Input: part model. Units: mm. Frame: model coordinates. Face numbers are marked on the shaded views. Coordinates: 2 decimals unless noted, no trailing zeros. Write each loop counter-clockwise with the first axis right and the second up, starting at its lowest first coordinate (ties: lowest second). Pieces come first, ordered by that corner, then holes.
1) Draft query along Z for the marked faces 1, 2, 3 and 4. Return one class per face: pulls with the +Z half, pulls with the -Z half, needs draft (parallel to the pull), parting line crosses it, or undercut.
2) Section query D-D (x = 35). Output: boundary loops of the cut face in (y, z), then the cut area to 3 significant figures.
3) Line query: L1, parallel to Z at x = 35, y = 0.2; L2, parallel to Z at x = -27, y = 10.5; L3, parallel to Z at x = -70, y = 0.6. Output: solid intervals per line, ascending.
4) Section query A-A (y = 16.75). Output: boundary loops of the cut face in (x, z), then the cut area to 3 significant figures.
5) Pin query (flat end, axial travel): pin 1 Ø4 at (x, z) = (-7, 0) entering from -Y; pin 2 Ø4 at (x, y) = (-23, 17) entering from +Z; pin 3 Ø0.5 at (x, y) = (-12.5, 0.5) entering from -Z; pin 4 Ø0.8 at (x, y) = (-20.5, 0.5) entering from +Z. Return the tip coordinate at first contact, or that it passes through.
6) Section query C-C (z = -40). Output: boundary loops of the cut face in (x, y), then the cut area to 3 significant figures.
7) Section query B-B (x = -7). Output: boundary loops of the cut face in (y, z), then the cut area to 3 significant figures.
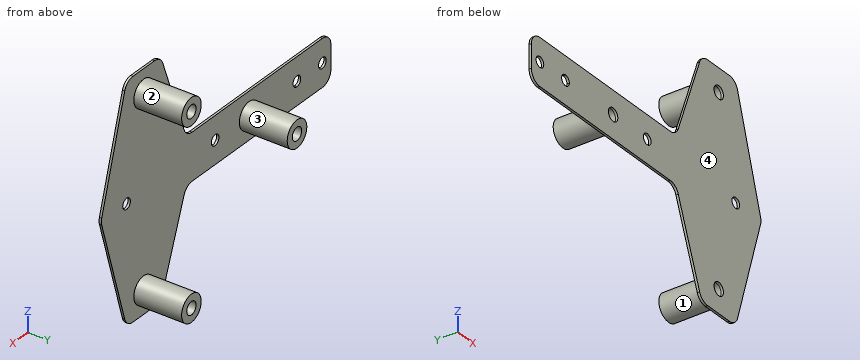
from build123d import *

# Parameters (mm, degrees)
BOSS_EXTRUDE1_DEPTH = 1
SKETCH2_R           = 2.75
CUT_EXTRUDE1_DEPTH  = 2
SKETCH3_R           = 5.75
SKETCH3_R_2         = 2.75
BOSS_EXTRUDE2_DEPTH = 20.5
SKETCH4_R           = 2.25
CUT_EXTRUDE2_DEPTH  = 2
SKETCH5_R           = 2.25
BOSS_EXTRUDE3_DEPTH = 1
SKETCH6_R           = 2.25
CUT_EXTRUDE3_DEPTH  = 2


with BuildPart() as part:
    # Sketch1 → Boss-Extrude1 (new body)
    with BuildSketch(Plane(origin=(0, 0, 0), x_dir=(1, 0, 0), z_dir=(0, 1, 0))):
        with BuildLine():
            Line((-55, 10), (6.534997659, 10))
            ThreePointArc((6.534997659, 10), (9.382971848, 10.890371912), (11.216643547, 13.244382792))
            Line((11.216643547, 13.244382792), (23.783356453, 46.755617208))
            ThreePointArc((23.783356453, 46.755617208), (25.617028152, 49.109628088), (28.465002341, 50))
            Line((28.465002341, 50), (41.279846746, 50))
            ThreePointArc((41.279846746, 50), (44.264499394, 49.011464641), (46.068978172, 46.436739428))
            Line((46.068978172, 46.436739428), (59.568978172, 1.436739428))
            ThreePointArc((59.568978172, 1.436739428), (59.779846746, 0), (59.568978172, -1.436739428))
            Line((59.568978172, -1.436739428), (46.068978172, -46.436739428))
            ThreePointArc((46.068978172, -46.436739428), (44.264499394, -49.011464641), (41.279846746, -50))
            Line((41.279846746, -50), (28.465002341, -50))
            ThreePointArc((28.465002341, -50), (25.617028152, -49.109628088), (23.783356453, -46.755617208))
            Line((23.783356453, -46.755617208), (11.216643547, -13.244382792))
            ThreePointArc((11.216643547, -13.244382792), (9.382971848, -10.890371912), (6.534997659, -10))
            Line((6.534997659, -10), (-55, -10))
            ThreePointArc((-55, -10), (-58.535533906, -8.535533906), (-60, -5))
            Line((-60, -5), (-60, 5))
            ThreePointArc((-60, 5), (-58.535533906, 8.535533906), (-55, 10))
        make_face()
    extrude(amount=BOSS_EXTRUDE1_DEPTH)

    # Sketch2 → Cut-Extrude1 (cut, through all)
    with BuildSketch(Plane(origin=(0, 1, 0), x_dir=(1, 0, 0), z_dir=(0, 1, 0))):
        with Locations((-27, 0)):
            Circle(SKETCH2_R)
        with Locations((35, 40)):
            Circle(SKETCH2_R)
        with Locations((35, -40)):
            Circle(SKETCH2_R)
    extrude(amount=-CUT_EXTRUDE1_DEPTH, mode=Mode.SUBTRACT)

    # Sketch3 → Boss-Extrude2 (add)
    with BuildSketch(Plane(origin=(0, 1, 0), x_dir=(1, 0, 0), z_dir=(0, 1, 0))):
        with Locations((-27, 0)):
            Circle(SKETCH3_R)
        with Locations((-27, 0)):
            Circle(SKETCH3_R_2, mode=Mode.SUBTRACT)
        with Locations((35, 40)):
            Circle(SKETCH3_R)
        with Locations((35, 40)):
            Circle(SKETCH3_R_2, mode=Mode.SUBTRACT)
        with Locations((35, -40)):
            Circle(SKETCH3_R)
        with Locations((35, -40)):
            Circle(SKETCH3_R_2, mode=Mode.SUBTRACT)
    extrude(amount=BOSS_EXTRUDE2_DEPTH)

    # Sketch4 → Cut-Extrude2 (cut, through all)
    with BuildSketch(Plane(origin=(0, 1, 0), x_dir=(1, 0, 0), z_dir=(0, 1, 0))):
        with Locations((-55, 0)):
            Circle(SKETCH4_R)
        with Locations((45, 0)):
            Circle(SKETCH4_R)
        with Locations((-7, 0)):
            Circle(SKETCH4_R)
    extrude(amount=-CUT_EXTRUDE2_DEPTH, mode=Mode.SUBTRACT)

    # Sketch5 → Boss-Extrude3 (add)
    with BuildSketch(Plane(origin=(0, 0, 0), x_dir=(1, 0, 0), z_dir=(0, 1, 0))):
        with BuildLine():
            Line((-55, 10), (-70, 10))
            ThreePointArc((-70, 10), (-73.535533906, 8.535533906), (-75, 5))
            Line((-75, 5), (-75, -5))
            ThreePointArc((-75, -5), (-73.535533906, -8.535533906), (-70, -10))
            Line((-70, -10), (-55, -10))
            Line((-55, -10), (-55, 10))
        make_face()
        with Locations((-70, 0)):
            Circle(SKETCH5_R, mode=Mode.SUBTRACT)
    extrude(amount=BOSS_EXTRUDE3_DEPTH)

    # Sketch6 → Cut-Extrude3 (cut, through all)
    with BuildSketch(Plane(origin=(0, 1, 0), x_dir=(1, 0, 0), z_dir=(0, 1, 0))):
        with Locations((-55, 0)):
            Circle(SKETCH6_R)
    extrude(amount=-CUT_EXTRUDE3_DEPTH, mode=Mode.SUBTRACT)


solid = part.part
Answer:
1. face 1: undercut
1. face 2: undercut
1. face 3: parting line crosses it
1. face 4: needs draft
2. outline: (0, -50) - (1, -50) - (1, -45.75) - (21.5, -45.75) - (21.5, -42.75) - (0, -42.75) - close; (0, -37.25) - (21.5, -37.25) - (21.5, -34.25) - (1, -34.25) - (1, 34.25) - (21.5, 34.25) - (21.5, 37.25) - (0, 37.25) - close; (0, 42.75) - (21.5, 42.75) - (21.5, 45.75) - (1, 45.75) - (1, 50) - (0, 50) - close
2. area: 335 mm2
3. L1: z = -50 to -42.75, -37.25 to 37.25, 42.75 to 50
3. L2: z = -5.75 to -2.75, 2.75 to 5.75
3. L3: z = -10 to -2.25, 2.25 to 10
4. outline: circle Ø11.5 at (-27, 0); circle Ø11.5 at (35, -40); circle Ø11.5 at (35, 40); hole circle Ø5.5 at (-27, 0); hole circle Ø5.5 at (35, -40); hole circle Ø5.5 at (35, 40)
4. area: 240 mm2
5. pin 1: passes through
5. pin 2: stops at z = 5.39
5. pin 3: stops at z = -10
5. pin 4: stops at z = 10
6. outline: (21.25, 0) - (32.25, 0) - (32.25, 21.5) - (29.25, 21.5) - (29.25, 1) - (21.25, 1) - close; (37.75, 0) - (48, 0) - (48, 1) - (40.75, 1) - (40.75, 21.5) - (37.75, 21.5) - close
6. area: 144 mm2
7. outline: (0, -10) - (1, -10) - (1, -2.25) - (0, -2.25) - close; (0, 2.25) - (1, 2.25) - (1, 10) - (0, 10) - close
7. area: 15.5 mm2
